The listing builds one solid part. Answer for the finished solid, in the listing's coordinates (mm). A direction names the side the tool comes from. Give positions to 0.01 mm unless a question says otherwise; leave off trailing zeros. Order: outer loops, then holes, each group sorted by start corner. A loop starts at its lowest first (then second) coordinate and runs counter-clockwise, first axis right, second up.
```python
from build123d import *

# Parameters (mm, degrees)
BOSS_EXTRUDE1_DEPTH = 88.9
SKETCH2_R           = 1.397
CUT_EXTRUDE1_DEPTH  = 100.443456884
SKETCH3_W           = 25.4
SKETCH3_H           = 5.08
CUT_EXTRUDE2_DEPTH  = 100.443456884
SKETCH5_W           = 25.4
SKETCH5_H           = 10.16
BOSS_EXTRUDE3_DEPTH = 3.81
SKETCH6_W           = 8.89
SKETCH6_H           = 63.5
CUT_EXTRUDE3_DEPTH  = 100.443456884


with BuildPart() as part:
    # Sketch1 → Boss-Extrude1 (new body)
    with BuildSketch(Plane.XY):
        Polygon((-40.203883769, 5.937788296), (40.203883769, 5.937788296), (44.399042974, 2.127788296), (-44.399042974, 2.127788296), align=None)
    extrude(amount=BOSS_EXTRUDE1_DEPTH)

    # Sketch2 → Cut-Extrude1 (cut, through all)
    with BuildSketch(Plane.XZ.offset(-2.127788296)):
        with Locations(Location((-31.369, 81.429995649, 0), (0, 0, 270))):
            Circle(SKETCH2_R)
        with Locations(Location((17.653, 23.517995649, 0), (0, 0, 270))):
            Circle(SKETCH2_R)
        with Locations(Location((-31.369, 23.517995649, 0), (0, 0, 270))):
            Circle(SKETCH2_R)
        with Locations(Location((17.653, 81.429995649, 0), (0, 0, 270))):
            Circle(SKETCH2_R)
    extrude(amount=-CUT_EXTRUDE1_DEPTH, mode=Mode.SUBTRACT)

    # Sketch3 → Cut-Extrude2 (cut, through all)
    with BuildSketch(Plane.XZ.offset(-2.127788296)):
        with Locations((0, 86.36)):
            Rectangle(SKETCH3_W, SKETCH3_H)
        with Locations((0, 2.54)):
            Rectangle(SKETCH3_W, SKETCH3_H)
    extrude(amount=-CUT_EXTRUDE2_DEPTH, mode=Mode.SUBTRACT)

    # Sketch5 → Boss-Extrude3 (add)
    with BuildSketch(Plane.XZ.offset(-2.127788296)):
        Rectangle(SKETCH5_W, SKETCH5_H)
    extrude(amount=-BOSS_EXTRUDE3_DEPTH)

    # Sketch6 → Cut-Extrude3 (cut, through all)
    with BuildSketch(Plane.XZ.offset(-2.127788296)):
        with Locations((32.334042974, 41.91)):
            Rectangle(SKETCH6_W, SKETCH6_H)
    extrude(amount=-CUT_EXTRUDE3_DEPTH, mode=Mode.SUBTRACT)


solid = part.part
```
1) Find section C-C (x = -1). Write down the section's boundary in (y, z), then the cut area to 3 significant figures.
Geometry says:
outline: (2.13, -5.08) - (5.94, -5.08) - (5.94, 83.82) - (2.13, 83.82) - close
area: 339 mm2
2) Find section B-B (y = 3.65). Write down the section's boundary in (x, z), then the cut area to 3 significant figures.
Geometry says:
outline: (-42.72, 0) - (-12.7, 0) - (-12.7, -5.08) - (12.7, -5.08) - (12.7, 0) - (42.72, 0) - (42.72, 88.9) - (12.7, 88.9) - (12.7, 83.82) - (-12.7, 83.82) - (-12.7, 88.9) - (-42.72, 88.9) - close; hole circle Ø2.79 at (-31.37, 23.52); hole circle Ø2.79 at (-31.37, 81.43); hole circle Ø2.79 at (17.65, 23.52); hole circle Ø2.79 at (17.65, 81.43); hole (27.89, 10.16) - (36.78, 10.16) - (36.78, 73.66) - (27.89, 73.66) - close
area: 7,010 mm2
3) Find section A-A (z = 36). Write down the section's boundary in (x, y), then the cut area to 3 significant figures.
Geometry says:
outline: (-44.4, 2.13) - (27.89, 2.13) - (27.89, 5.94) - (-40.2, 5.94) - close; (36.78, 2.13) - (44.4, 2.13) - (40.2, 5.94) - (36.78, 5.94) - close
area: 288 mm2
4) For a pull along X with two mould halves and no side action, classify faces 4 (the flat face through (42.27, 4.06, 43.83)), 5 (the flat face through (-28, 4, 0)), 6 (the flat face through (-12.7, 4, -3)), 7 (the flat face through (-12.7, 4, 86)) as +X half, -X half, draft (parallel to the pull), parting line (faces both ways), or undercut.
Geometry says:
face 4: +X half
face 5: draft
face 6: -X half
face 7: undercut
5) Straight lines are drawn through the part: probe 1 along Z at (x, y) = (35, 4.45); probe 2 along Z at (x, y) = (-41, 2.9); probe 3 along X at (y, z) = (4.8, 20.5). For each, find the intervals that lie inside material, in ascending order.
Geometry says:
probe 1: z = 0 to 10.16, 73.66 to 88.9
probe 2: z = 0 to 88.9
probe 3: x = -41.46 to 27.89, 36.78 to 41.46
6) Given P1, Ø1.1, axis at y = 4.5, z = -2, coming from the -X side; P2, Ø1.1, axis at x = 33, y = 4, coming from the -Z side, each flat-ended and moving along its own axis, determine where each tip first touches the part or whether it passes through.
Geometry says:
P1: stops at x = -12.7
P2: stops at z = 0
7) A tool of negligible diameter and unlimited length cuts with its end or side. For faces 1 (the flat face through (32, 4, 73.66)), 2 (the flat face through (29, 4, 0)), 3 (the flat face through (0, 4, 83.82)), from which of +Z, -Z, +X, -X, +Y, -Y can it reach the whole face along a straight path? Write none if from no direction.
Geometry says:
face 1: +Y, -Y
face 2: -Z, +X, +Y, -Y
face 3: +Z, +Y, -Y
